Verification items for this drawing (mm, ordinates from the low corner). A direction names the side the tool comes from. Round coordinates to 2 decimals unless told otherwise and drop trailing zeros. Loops run counter-clockwise (first coordinate to the right, second up) from the corner with the lowest first, then second, coordinate; pieces in that order, holes last. Notation, with made-up numbers: M 45,-28 L 85,-28 A23 cw 85,-9 Z; hole C 88.25,69 d10. An arc over 180 degrees is marked long. Write item = value, one per line. Start each with the question number.
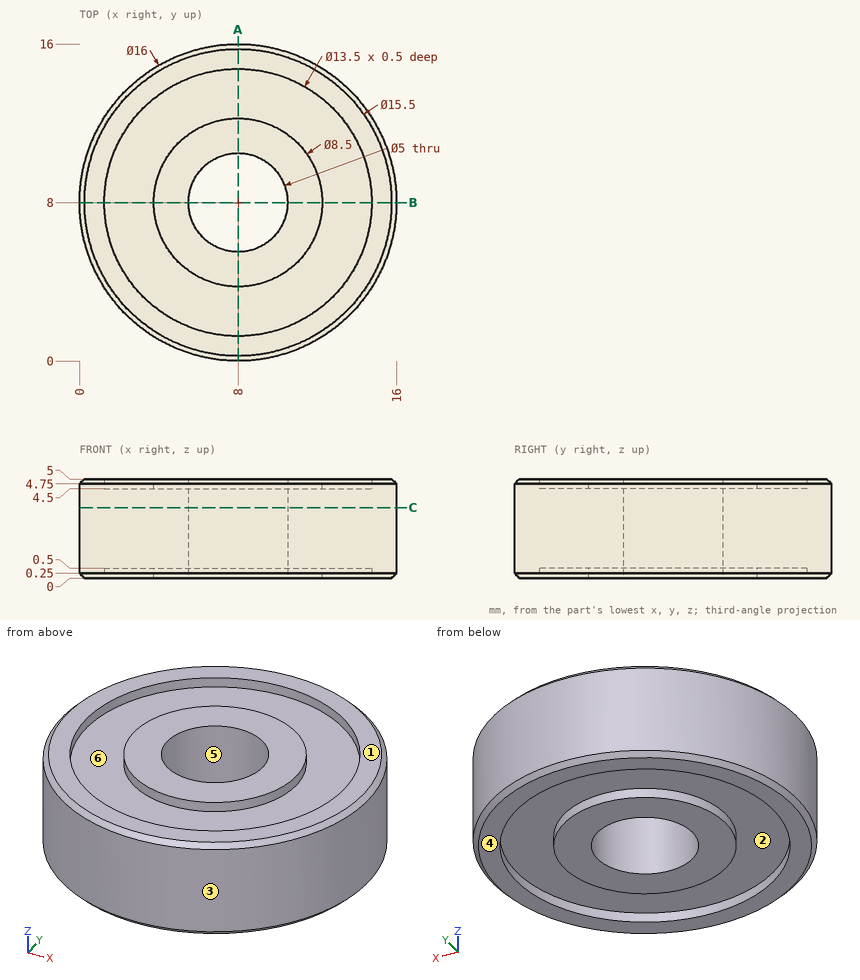
1. Tool access check on the marked faces 1 and 2. Record the directions out of +Z, -Z, +X, -X, +Y, -Y that give a thin tool (end or side, any length) a straight path to the whole face; none if there is none.
2. Thickness scan on line 1 (Y direction, x = 8, z = 0.35); line 2 (Y direction, x = 8, z = 4.8); line 3 (Y direction, x = 8, z = 2.55). Record the ranges inside material, lowest first.
3. Mould release check, pull along X, two halves, no side actions. Record for the marked faces 3, 4, 5 and 6: pulls with the +X half, pulls with the -X half, needs draft (parallel to the pull), parting line crosses it, or undercut.
4. Gauge pin test, flat ends, axial feed: P1, Ø3, axis at x = 5.5, z = 4, coming from the +Y side; P2, Ø1.5, axis at y = 13.5, z = 2.5, coming from the +X side; P3, Ø3, axis at x = 14.5, z = 1, coming from the +Y side (3 decimals). Record the tip position at first contact, or that the pin passes through.
5. Section check C-C, the plane z = 3.55. Enter the section's corners in (x, y), and give its area (3 significant figures).
6. Section check A-A, the plane x = 8. Enter the section's corners in (y, z), and give its area (3 significant figures).
Computed values:
q1.face_1 = +Z, +X, -X, +Y, -Y
q1.face_2 = -Z
q2.line_1 = 0 to 1.25, 3.75 to 5.5, 10.5 to 12.25, 14.75 to 16
q2.line_2 = 0.05 to 1.25, 3.75 to 5.5, 10.5 to 12.25, 14.75 to 15.95
q2.line_3 = 0 to 5.5, 10.5 to 16
q3.face_3 = parting line crosses it
q3.face_4 = needs draft
q3.face_5 = undercut
q3.face_6 = undercut
q4.P1 = 15.94
q4.P2 = 14.44
q4.P3 = 14.245
q5.outline = C 8,8 d16; hole C 8,8 d5
q5.area = 181 mm2
q6.outline = M 0,0.25 L 0.25,0 L 1.25,0 L 1.25,0.5 L 3.75,0.5 L 3.75,0 L 5.5,0 L 5.5,5 L 3.75,5 L 3.75,4.5 L 1.25,4.5 L 1.25,5 L 0.25,5 L 0,4.75 Z; M 10.5,0 L 12.25,0 L 12.25,0.5 L 14.75,0.5 L 14.75,0 L 15.75,0 L 16,0.25 L 16,4.75 L 15.75,5 L 14.75,5 L 14.75,4.5 L 12.25,4.5 L 12.25,5 L 10.5,5 Z
q6.area = 49.9 mm2
